CAD build for the part. Positions are in the model's coordinates, mm. Face numbers are marked on the shaded views. A direction names the side the tool comes from. Round coordinates to 2 decimals unless told otherwise and drop trailing zeros. Write each loop counter-clockwise with the first axis right and the second up, starting at its lowest first coordinate (ties: lowest second). Pieces come first, ordered by that corner, then holes. Notation, with made-up numbers: (-15.75, 48) - (3.25, 48) arc R20 ccw to (3.25, 53) - close; hole circle Ø7 at (-3, 49). An arc over 180 degrees is marked (long way). Answer in a Markdown table with one row per item.
```python
from build123d import *

# Parameters (mm, degrees)
SKETCH1_R                     = 43.815
HOUSING_FITTING_EXTRUDE_DEPTH = 17.018
HOUSING_BODY_1_DEPTH          = 22.6822
SKETCH3_R                     = 6.731
IMPELLER_BORE_DEPTH           = 17.018
SKETCH4_R                     = 4
SHAFT_BORE_DEPTH              = 70.612
O_RING_CUT_DEPTH              = 1.27
O_RING_CUT_DEPTH_BACK         = 3.175
SKETCH5_R                     = 43.942
SKETCH5_R_2                   = 41.402
SKETCH12_R                    = 3.175
CUT_EXTRUDE2_DEPTH            = 19.05
CIRPATTERN1_COUNT             = 8
SKETCH14_R                    = 3.175
SKETCH14_R_2                  = 3.392842108
CUT_EXTRUDE4_DEPTH            = 16.51
SKETCH15_R                    = 3.175
CUT_EXTRUDE5_DEPTH            = 10.922
FILLET1_R                     = 6.604
SKETCH16_R                    = 11.811
CUT_EXTRUDE7_DEPTH            = 32.0929
SKETCH17_R                    = 19.558
CUT_EXTRUDE8_DEPTH            = 13.0429


with BuildPart() as part:
    # Sketch1 → Housing Fitting Extrude (new body)
    with BuildSketch(Plane(origin=(0, 0, 0), x_dir=(0, 0, -1), z_dir=(1, 0, 0))):
        Circle(SKETCH1_R)
    extrude(amount=HOUSING_FITTING_EXTRUDE_DEPTH)

    # Sketch2 → Housing Body 1 (add)
    with BuildSketch(Plane.ZY):
        with BuildLine():
            Line((60.96, 0), (60.96, 60.96))
            Line((60.96, 60.96), (0, 60.96))
            ThreePointArc((0, 60.96), (-43.105229381, 43.105229381), (-60.96, 0))
            Line((-60.96, 0), (-60.96, -54.61))
            Line((-60.96, -54.61), (-60.96, -60.96))
            Line((-60.96, -60.96), (60.96, -60.96))
            Line((60.96, -60.96), (60.96, -54.61))
            Line((60.96, -54.61), (60.96, 0))
        make_face()
    extrude(amount=HOUSING_BODY_1_DEPTH)

    # Sketch3 → Impeller Bore (cut)
    with BuildSketch(Plane(origin=(17.018, 0, 0), x_dir=(0, 0, -1), z_dir=(1, 0, 0))):
        Circle(SKETCH3_R)
    extrude(amount=-IMPELLER_BORE_DEPTH, mode=Mode.SUBTRACT)

    # Sketch4 → Shaft Bore (cut)
    with BuildSketch(Plane(origin=(0, 0, 0), x_dir=(0, 0, -1), z_dir=(1, 0, 0))):
        Circle(SKETCH4_R)
    extrude(amount=-SHAFT_BORE_DEPTH, mode=Mode.SUBTRACT)

    # Sketch5 → O-Ring Cut (cut, two sides: drawn at the far end of the back side and taken through both)
    with BuildSketch(Plane(origin=(8.509, 0, 0), x_dir=(0, 0, -1), z_dir=(1, 0, 0)).offset(-O_RING_CUT_DEPTH_BACK)):
        Circle(SKETCH5_R)
        Circle(SKETCH5_R_2, mode=Mode.SUBTRACT)
    extrude(amount=O_RING_CUT_DEPTH + O_RING_CUT_DEPTH_BACK, mode=Mode.SUBTRACT)

    # Sketch12 → Cut-Extrude2 (cut)
    with BuildSketch(Plane(origin=(0, 0, 0), x_dir=(0, 0, -1), z_dir=(1, 0, 0))):
        with Locations((-50.419, 0)):
            Circle(SKETCH12_R)
    cut_extrude2 = extrude(amount=-CUT_EXTRUDE2_DEPTH, mode=Mode.SUBTRACT)

    # CirPattern1: Cut-Extrude2 ×8 about axis, 1 skipped
    cirpattern1_axis = Axis((0, 0, 0), (1, 0, 0))
    add([cut_extrude2.rotate(cirpattern1_axis, i * 360 / CIRPATTERN1_COUNT) for i in range(1, CIRPATTERN1_COUNT) if i not in (7,)], mode=Mode.SUBTRACT)

    # Sketch14 → Cut-Extrude4 (cut)
    with BuildSketch(Plane.XZ.offset(60.96)):
        with Locations(Location((-9.525, -46.754349092, 0), (0, 0, 270))):
            Circle(SKETCH14_R)
        with Locations(Location((-9.525, 41.914080666, 0), (0, 0, 270))):
            Circle(SKETCH14_R_2)
    extrude(amount=-CUT_EXTRUDE4_DEPTH, mode=Mode.SUBTRACT)

    # Sketch15 → Cut-Extrude5 (cut)
    with BuildSketch(Plane(origin=(0, 0, -60.96), x_dir=(-1, 0, 0), z_dir=(0, 0, -1))):
        with Locations(Location((9.525, -39.337514031, 0), (0, 0, 90))):
            Circle(SKETCH15_R)
    extrude(amount=-CUT_EXTRUDE5_DEPTH, mode=Mode.SUBTRACT)

    # Fillet1
    fillet1_edges = [part.edges().sort_by_distance(p)[0] for p in [
        (17.018, 0, 6.731),
    ]]
    fillet(fillet1_edges, radius=FILLET1_R)

    # Sketch16 → Cut-Extrude7 (cut)
    with BuildSketch(Plane.ZY.offset(22.6822)):
        Circle(SKETCH16_R)
    extrude(amount=-CUT_EXTRUDE7_DEPTH, mode=Mode.SUBTRACT)

    # Sketch17 → Cut-Extrude8 (cut)
    with BuildSketch(Plane.ZY.offset(22.6822)):
        Circle(SKETCH17_R)
    extrude(amount=-CUT_EXTRUDE8_DEPTH, mode=Mode.SUBTRACT)


solid = part.part
```
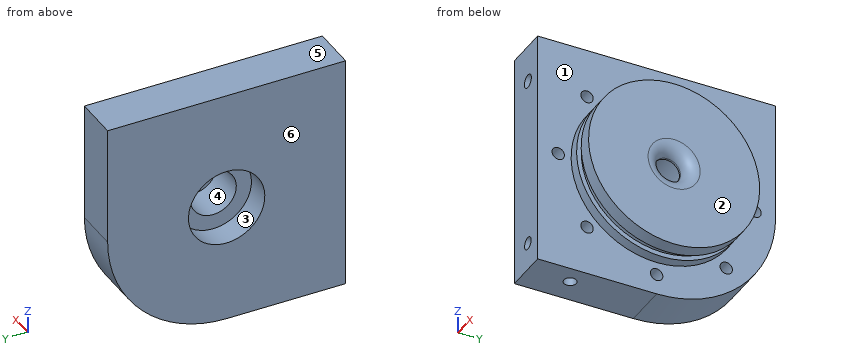
Q1. 3-axis set-ups, long thin cutter, end or side, ignore diameter. For the marked faces 1, 2 and 3: which of +Z, -Z, +X, -X, +Y, -Y reach the whole face in a straight line?
Computed:
| item | result |
|---|---|
| face 1 | +X |
| face 2 | +Z, -Z, +X, +Y, -Y |
| face 3 | -X |
Q2. Drill centre lines: line 1 (Y direction, x = -4.5, z = 2); line 2 (Z direction, x = 13, y = -2.5); line 3 (X direction, y = -1, z = -16.5). Where is each one in solid material? Low to high.
Computed:
| item | result |
|---|---|
| line 1 | y = -60.96 to -52.88, -47.95 to -11.64, 11.64 to 47.95, 52.88 to 60.96 |
| line 2 | z = -43.74 to -6.81, 6.81 to 43.74 |
| line 3 | x = -9.64 to 17.02 |
Q3. Saw through at A-A on x = -17.5. Count the separate pieces of the cut face and the enclosed holes in it, then the cut area to 3 significant figures.
Computed:
| item | result |
|---|---|
| separate pieces | 1 |
| enclosed holes | 8 |
| area | 12,600 mm2 |
Q4. Saw through at C-C on z = -27. List the corners of the cut face in (x, y), then the cut area to 3 significant figures.
Computed:
| item | result |
|---|---|
| outline | (-22.68, -60.96) - (0, -60.96) - (0, -34.51) - (5.33, -34.51) - (5.33, -31.39) - (9.78, -31.39) - (9.78, -34.51) - (17.02, -34.51) - (17.02, 34.51) - (9.78, 34.51) - (9.78, 31.39) - (5.33, 31.39) - (5.33, 34.51) - (0, 34.51) - (0, 54.65) - (-22.68, 54.65) - close |
| area | 3,770 mm2 |
Q5. Flat gauge pins, fed straight in: pin 1 (8.5 mm diameter, centred on y = -35.65, z = -35.65, fed in from +X); pin 2 (1.9 mm diameter, centred on y = -34, z = -35, fed in from +X); pin 3 (3 mm diameter, centred on x = -8.5, y = -39, fed in from -Z); pin 4 (11 mm diameter, centred on y = 0, z = 0, fed in from -X). Where does each tip first touch, or does it go through?
Computed:
| item | result |
|---|---|
| pin 1 | stops at x = 0 |
| pin 2 | stops at x = -19.05 |
| pin 3 | stops at z = -50.04 |
| pin 4 | passes through |
Q6. Saw through at B-B on y = -30.5. List the corners of the cut face in (x, z).
Computed:
| item | result |
|---|---|
| outline | (-22.68, -60.96) - (0, -60.96) - (0, -31.46) - (5.33, -31.46) - (5.33, -28) - (9.78, -28) - (9.78, -31.46) - (17.02, -31.46) - (17.02, 31.46) - (9.78, 31.46) - (9.78, 28) - (5.33, 28) - (5.33, 31.46) - (0, 31.46) - (0, 60.96) - (-22.68, 60.96) - close |
Q7. Pull direction Z, two halves, no side cores. Call the marked faces 4, 5 and 6: released by +Z, released by -Z, zero draft, split by the parting line, or undercut.
Computed:
| item | result |
|---|---|
| face 4 | undercut |
| face 5 | released by +Z |
| face 6 | zero draft |
Q8. Saw through at D-D on x = 13. List the corners of the cut face in (y, z) (3 decimals), then the cut area to 3 significant figures.
Computed:
| item | result |
|---|---|
| outline | circle Ø87.63 at (0, 0); hole circle Ø14.517 at (0, 0) |
| area | 5,870 mm2 |
